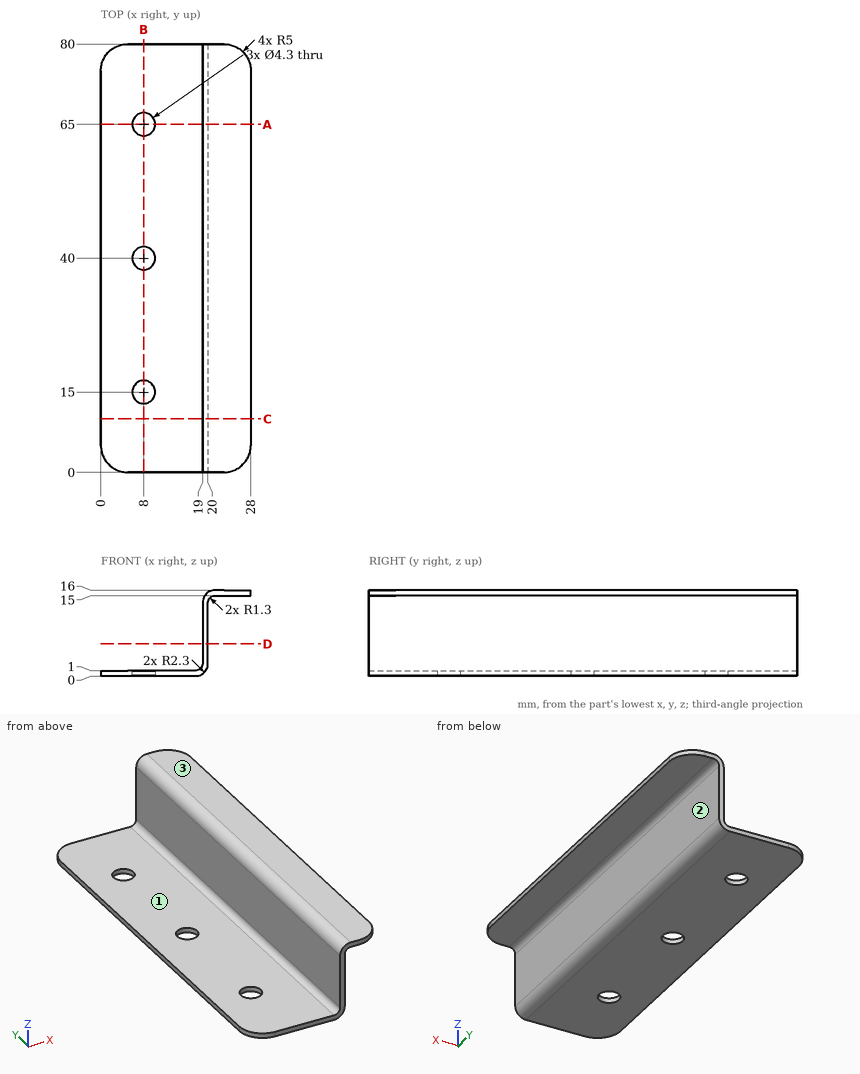
Answer from the drawing. Dimensions are ordinates in mm from the lowest x, y and z of the part. A direction names the side the tool comes from. Give positions to 0.01 mm unless a question says otherwise; leave off trailing zeros. Order: outer loops, then holes, each group sorted by start corner. A loop starts at its lowest first (then second) coordinate and runs counter-clockwise, first axis right, second up.
(1) Straight lines are drawn through the part: L1, parallel to Y at x = 8, z = 0.25; L2, parallel to Z at x = 9.5, y = 34.5; L3, parallel to X at y = 45.5, z = 11.25. For each, find the intervals that lie inside material, in ascending order.
(2) For the marked faces 1, 2 and 3, determine the directions among +Z, -Z, +X, -X, +Y, -Y from which every point of the face is accessible in a straight line to the end or side of a thin tool.
(3) Find section B-B (x = 8). Give the vertices of the cut face in (y, z), plus the area to 3 significant figures.
(4) Find section C-C (y = 10). Give the vertices of the cut face in (x, z).
(5) Find section D-D (z = 6). Give the vertices of the cut face in (x, y), plus the area to 3 significant figures.
(6) Find section A-A (y = 65). Give the vertices of the cut face in (x, z).
(7) Given pin 1 (5.5 mm diameter, centred on x = 26, y = 42, fed in from -Z); pin 2 (3 mm diameter, centred on x = 19.5, y = 52, fed in from +Z); pin 3 (7 mm diameter, centred on x = 8, y = 40, fed in from +Z); pin 4 (3 mm diameter, centred on x = 19, y = 56.5, fed in from -Z), each flat-ended and moving along its own axis, determine where each tip first touches the part or whether it passes through.
Result sheet:
1. L1: y = 0 to 12.85, 17.15 to 37.85, 42.15 to 62.85, 67.15 to 80
1. L2: z = 0 to 1
1. L3: x = 19 to 20
2. face 1: +Z, -X, +Y, -Y
2. face 2: -Z, +X, +Y, -Y
2. face 3: +Z, +X, -X, +Y, -Y
3. outline: (0, 0) - (12.85, 0) - (12.85, 1) - (0, 1) - close; (17.15, 0) - (37.85, 0) - (37.85, 1) - (17.15, 1) - close; (42.15, 0) - (62.85, 0) - (62.85, 1) - (42.15, 1) - close; (67.15, 0) - (80, 0) - (80, 1) - (67.15, 1) - close
3. area: 67.1 mm2
4. outline: (0, 0) - (17.7, 0) arc R2.3 ccw to (20, 2.3) - (20, 13.7) arc R1.3 cw to (21.3, 15) - (28, 15) - (28, 16) - (21.3, 16) arc R2.3 ccw to (19, 13.7) - (19, 2.3) arc R1.3 cw to (17.7, 1) - (0, 1) - close
5. outline: (19, 0) - (20, 0) - (20, 80) - (19, 80) - close
5. area: 80.0 mm2
6. outline: (0, 0) - (5.85, 0) - (5.85, 1) - (0, 1) - close; (10.15, 0) - (17.7, 0) arc R2.3 ccw to (20, 2.3) - (20, 13.7) arc R1.3 cw to (21.3, 15) - (28, 15) - (28, 16) - (21.3, 16) arc R2.3 ccw to (19, 13.7) - (19, 2.3) arc R1.3 cw to (17.7, 1) - (10.15, 1) - close
7. pin 1: stops at z = 15
7. pin 2: stops at z = 15.98
7. pin 3: stops at z = 1
7. pin 4: stops at z = 0
